Part model, mm, in its own coordinate system. Round coordinates to 2 decimals unless told otherwise and drop trailing zeros. Write each loop counter-clockwise with the first axis right and the second up, starting at its lowest first coordinate (ties: lowest second). Pieces come first, ordered by that corner, then holes.
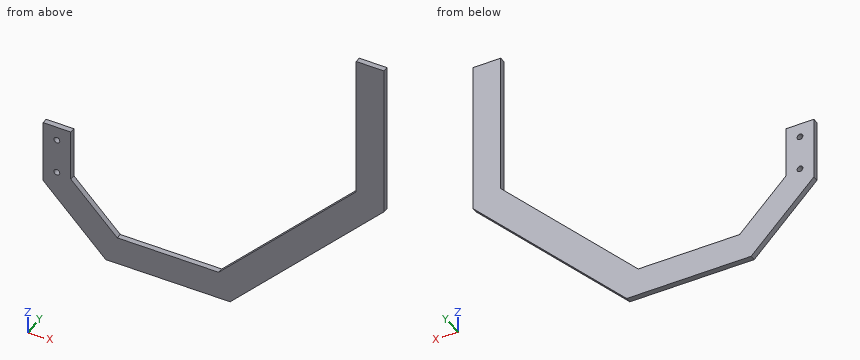
```python
from build123d import *

# Parameters (mm, degrees)
SKETCH_1_R      = 2.1
EXTRUDE_1_DEPTH = 4


with BuildPart() as part:
    # 草图1 → 凸台-拉伸1 (new body)
    with BuildSketch(Plane(origin=(0, 0, 0), x_dir=(1, 0, 0), z_dir=(0, 1, 0))):
        Polygon((20, 0), (0, 0), (0, 45), (45.25, 90.25), (134.96758269, 90.25), (245.824430246, -20.606847556), (245.824430246, -130.606847556), (225.824430246, -130.606847556), (225.824430246, -28.891118804), (126.683311442, 70.25), (53.534271247, 70.25), (20, 36.715728753), align=None)
        with Locations(Location((10, 10, 0), (0, 0, 270))):
            Circle(SKETCH_1_R, mode=Mode.SUBTRACT)
        with Locations(Location((10, 35, 0), (0, 0, 90))):
            Circle(SKETCH_1_R, mode=Mode.SUBTRACT)
    extrude(amount=EXTRUDE_1_DEPTH)


solid = part.part
```
Q1. Wall check: L1, parallel to X at y = 1.05, z = -35; L2, parallel to X at y = 1.5, z = -10; L3, parallel to X at y = 3, z = 57.5. Give the ranges that are in metal, low to high.
Values follow:
L1: x = 0 to 7.9, 12.1 to 20, 161.93 to 190.22
L2: x = 0 to 7.9, 12.1 to 20, 186.93 to 215.22
L3: x = 225.82 to 245.82
Q2. Cut at D-D on x = 160. Write the cut outline in (y, z).
Values follow:
outline: (0, -65.22) - (4, -65.22) - (4, -36.93) - (0, -36.93) - close
Q3. Drop flat-ended pins along their axis: pin 1 (2 mm diameter, centred on x = 103, y = 2.5, fed in from +Z); pin 2 (5.5 mm diameter, centred on x = 10, z = -10, fed in from +Y); pin 3 (1.2 mm diameter, centred on x = 7, y = 2, fed in from +Z); pin 4 (1.2 mm diameter, centred on y = 2.5, z = -15, fed in from +X). Give the stop position or say it passes through.
Values follow:
pin 1: stops at z = -70.25
pin 2: stops at y = 4
pin 3: stops at z = 0
pin 4: stops at x = 210.82
Q4. Cut at B-B on z = -20.5. Write the cut outline in (x, y).
Values follow:
outline: (0, 0) - (20, 0) - (20, 4) - (0, 4) - close; (176.43, 0) - (204.72, 0) - (204.72, 4) - (176.43, 4) - close
Q5. Cut at A-A on y = 1.05. Write the cut outline in (x, z), plus the area to 3 significant figures.
Values follow:
outline: (0, -45) - (45.25, -90.25) - (134.97, -90.25) - (245.82, 20.61) - (245.82, 130.61) - (225.82, 130.61) - (225.82, 28.89) - (126.68, -70.25) - (53.53, -70.25) - (20, -36.72) - (20, 0) - (0, 0) - close; hole circle Ø4.2 at (10, -35); hole circle Ø4.2 at (10, -10)
area: 8,620 mm2
Q6. Cut at C-C on z = 83. Write the cut outline in (x, y).
Values follow:
outline: (225.82, 0) - (245.82, 0) - (245.82, 4) - (225.82, 4) - close
